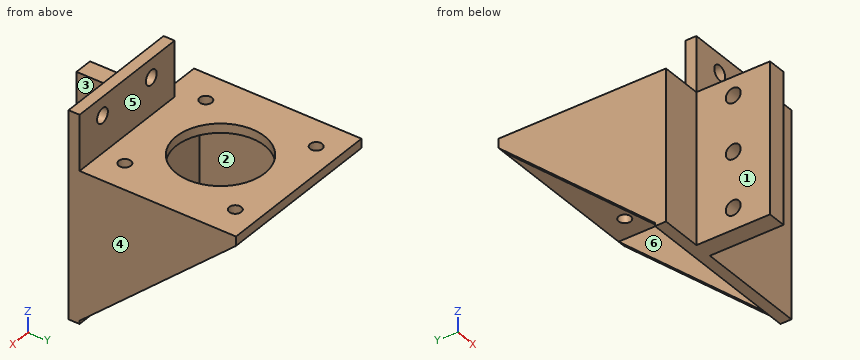
```python
from build123d import *

# Parameters (mm, degrees)
SKETCH1_R           = 2
BOSS_EXTRUDE1_DEPTH = 3
BOSS_EXTRUDE2_DEPTH = 42.5
CUT_EXTRUDE1_DEPTH  = 77.832667384
SKETCH4_R           = 12
SKETCH4_R_2         = 1.65
CUT_EXTRUDE2_DEPTH  = 82.92227278
SKETCH6_W           = 5
SKETCH6_H           = 40.874916237
BOSS_EXTRUDE3_DEPTH = 20
SKETCH7_R           = 2.025
CUT_EXTRUDE4_DEPTH  = 69.231144603


with BuildPart() as part:
    # Sketch1 → Boss-Extrude1 (new body)
    with BuildSketch(Plane(origin=(0, 0, 0), x_dir=(1, 0, 0), z_dir=(0, 1, 0))):
        Polygon((54.5, 0.874916237), (54.5, 40.874916237), (8, 40.874916237), (8, 0), (19.259624399, 0), (19.259624399, -15), (54.5, -15), align=None)
        with Locations(Location((27.904171313, -10, 0), (0, 0, 270))):
            Circle(SKETCH1_R, mode=Mode.SUBTRACT)
        with Locations(Location((46.009358787, -10, 0), (0, 0, 270))):
            Circle(SKETCH1_R, mode=Mode.SUBTRACT)
    extrude(amount=BOSS_EXTRUDE1_DEPTH)

    # Sketch2 → Boss-Extrude2 (add)
    with BuildSketch(Plane(origin=(0, 3, 0), x_dir=(1, 0, 0), z_dir=(0, 1, 0))):
        Polygon((10, 2.5), (10, 40), (8, 40), (8, 0), (54.5, 0), (54.5, 40), (52.5, 40), (52.5, 2.5), align=None)
    extrude(amount=BOSS_EXTRUDE2_DEPTH)

    # Sketch3 → Cut-Extrude1 (cut, through all)
    with BuildSketch(Plane(origin=(54.5, 0, 0), x_dir=(0, 0, -1), z_dir=(1, 0, 0))):
        Polygon((40, 45.5), (2.5, 45.5), (40, 3), align=None)
    extrude(amount=-CUT_EXTRUDE1_DEPTH, mode=Mode.SUBTRACT)

    # Sketch4 → Cut-Extrude2 (cut, through all)
    with BuildSketch(Plane.XY):
        with Locations((31.25, 24.25)):
            Circle(SKETCH4_R)
        with Locations((16.25, 9.25)):
            Circle(SKETCH4_R_2)
        with Locations((16.25, 39.25)):
            Circle(SKETCH4_R_2)
        with Locations((46.25, 39.25)):
            Circle(SKETCH4_R_2)
        with Locations((46.25, 9.25)):
            Circle(SKETCH4_R_2)
    extrude(amount=-CUT_EXTRUDE2_DEPTH, mode=Mode.SUBTRACT)

    # Sketch6 → Boss-Extrude3 (add)
    with BuildSketch(Plane.XZ):
        with Locations((21.759624399, -20.437458119)):
            Rectangle(SKETCH6_W, SKETCH6_H)
    extrude(amount=BOSS_EXTRUDE3_DEPTH)

    # Sketch7 → Cut-Extrude4 (cut, through all)
    with BuildSketch(Plane(origin=(24.259624399, 0, 0), x_dir=(0, 0, -1), z_dir=(1, 0, 0))):
        with Locations((35, -10)):
            Circle(SKETCH7_R)
        with Locations((20, -10)):
            Circle(SKETCH7_R)
        with Locations((5, -10)):
            Circle(SKETCH7_R)
    extrude(amount=-CUT_EXTRUDE4_DEPTH, mode=Mode.SUBTRACT)


solid = part.part
```
Check sheet for the modelled part. Datum: model origin and axes. Units: mm. Face numbers are marked on the shaded views. A direction names the side the tool comes from. Round coordinates to 2 decimals unless told otherwise and drop trailing zeros. Write each loop counter-clockwise with the first axis right and the second up, starting at its lowest first coordinate (ties: lowest second). Pieces come first, ordered by that corner, then holes. Notation, with made-up numbers: (67.25, 52) -> (98.25, 52) arc R33 ccw to (98.25, 87) -> close; hole circle Ø5 at (89.5, 61.25). An arc over 180 degrees is marked (long way). Put each result on its own line as item: value.
(1) Sectioned sample at C-C (y = -10). Enter the section's corners in (x, z) (3 decimals), plus the area to 3 significant figures.
Values found:
outline: (19.26, -40.875) -> (24.26, -40.875) -> (24.26, -37.025) -> (19.26, -37.025) -> close; (19.26, -32.975) -> (24.26, -32.975) -> (24.26, -22.025) -> (19.26, -22.025) -> close; (19.26, -17.975) -> (24.26, -17.975) -> (24.26, -7.025) -> (19.26, -7.025) -> close; (19.26, -2.975) -> (24.26, -2.975) -> (24.26, 0) -> (19.26, 0) -> close
area: 144 mm^2
(2) Go/stop test with flat-tipped pins: pin 1 Ø10 at (x, z) = (41.5, -22.5) entering from +Y; pin 2 Ø6 at (y, z) = (36, -11) entering from +X; pin 3 Ø5.5 at (y, z) = (-10, -5) entering from -X; pin 4 Ø4.5 at (x, y) = (16.25, 39.25) entering from +Z. Record where each tip stops, or that it passes through.
Values found:
pin 1: stops at y = 3
pin 2: stops at x = 54.5
pin 3: stops at x = 19.26
pin 4: stops at z = 0
(3) Mould release check, pull along X, two halves, no side actions. Record for the marked faces 4, 5 and 6: released by +X, released by -X, zero draft, split by the parting line, or undercut.
Values found:
face 4: released by +X
face 5: zero draft
face 6: undercut
(4) Sectioned sample at A-A (y = 24.25). Enter the section's corners in (x, z), plus the area to 3 significant figures.
Values found:
outline: (8, -21.25) -> (10, -21.25) -> (10, -2.5) -> (19.25, -2.5) -> (19.25, 0) -> (8, 0) -> close; (43.25, -2.5) -> (52.5, -2.5) -> (52.5, -21.25) -> (54.5, -21.25) -> (54.5, 0) -> (43.25, 0) -> close
area: 131 mm^2
(5) Tool access check on the marked faces 1, 2 and 3. Record the directions out of +Z, -Z, +X, -X, +Y, -Y that give a thin tool (end or side, any length) a straight path to the whole face; none if there is none.
Values found:
face 1: +Z, -Z, -X, -Y
face 2: -Z, +Y
face 3: +Z, -Z, +X, -Y
(6) Sectioned sample at B-B (z = 10). Enter the section's corners in (x, y).
Values found:
outline: (19.26, 0) -> (25.9, 0) -> (25.9, 3) -> (19.26, 3) -> close; (29.9, 0) -> (44.01, 0) -> (44.01, 3) -> (29.9, 3) -> close; (48.01, 0) -> (54.5, 0) -> (54.5, 3) -> (48.01, 3) -> close
(7) Material ranges on line 1 (Y direction, x = 16.25, z = -1.55); line 2 (X direction, y = 9, z = -1); line 3 (X direction, y = 11, z = -24), recorded low to high.
Values found:
line 1: y = 0 to 7.6, 10.9 to 37.6, 40.9 to 45.5
line 2: x = 8 to 14.62, 17.88 to 44.62, 47.88 to 54.5
line 3: x = 8 to 10, 52.5 to 54.5
(8) Sectioned sample at D-D (z = -35). Enter the section's corners in (x, y) (3 decimals).
Values found:
outline: (8, 0) -> (19.26, 0) -> (19.26, -7.975) -> (24.26, -7.975) -> (24.26, 0) -> (54.5, 0) -> (54.5, 8.667) -> (52.5, 8.667) -> (52.5, 3) -> (10, 3) -> (10, 8.667) -> (8, 8.667) -> close; (19.26, -20) -> (24.26, -20) -> (24.26, -12.025) -> (19.26, -12.025) -> close
